```python
from build123d import *

# Parameters (mm, degrees)
SKETCH1_R           = 18.5
SKETCH1_R_2         = 11
BOSS_EXTRUDE1_DEPTH = 3.5
SKETCH2_R           = 4
CUT_EXTRUDE3_DEPTH  = 6.4
CIRPATTERN1_COUNT   = 6
SKETCH3_R           = 4.05
BOSS_EXTRUDE2_DEPTH = 6


with BuildPart() as part:
    # Sketch1 → Boss-Extrude1 (new body, symmetric)
    with BuildSketch(Plane.XY):
        Circle(SKETCH1_R)
        Circle(SKETCH1_R_2, mode=Mode.SUBTRACT)
    extrude(amount=BOSS_EXTRUDE1_DEPTH, both=True)

    # Sketch2 → Cut-Extrude3 (cut)
    with BuildSketch(Plane(origin=(-18.5, -17.193061184, 0), x_dir=(0, -1, 0), z_dir=(1, 0, 0))):
        with Locations((-17.193061184, 0)):
            Circle(SKETCH2_R)
    cut_extrude3 = extrude(amount=CUT_EXTRUDE3_DEPTH, mode=Mode.SUBTRACT)

    # CirPattern1: Cut-Extrude3 ×6 about axis
    cirpattern1_axis = Axis((0, 0, 0), (0, 0, 1))
    for i in range(1, CIRPATTERN1_COUNT):
        add(cut_extrude3.rotate(cirpattern1_axis, i * 360 / CIRPATTERN1_COUNT), mode=Mode.SUBTRACT)

    # Sketch3 → Boss-Extrude2 (add)
    with BuildSketch(Plane(origin=(-12.1, 0, 0), x_dir=(0, -1, 0), z_dir=(-1, 0, 0))):
        Circle(SKETCH3_R)
    extrude(amount=BOSS_EXTRUDE2_DEPTH)


solid = part.part
```
Check sheet for the modelled part. Datum: model origin and axes. Units: mm. A direction names the side the tool comes from. Coordinates: 2 decimals unless noted, no trailing zeros. Write each loop counter-clockwise with the first axis right and the second up, starting at its lowest first coordinate (ties: lowest second). Pieces come first, ordered by that corner, then holes. Notation, with made-up numbers: M 23.5,62 L 79.5,62 A9 cw 79.5,78 Z; hole C 48,20 d7. An arc over 180 degrees is marked long. Use one line per item in the form item = value.
Item 1: Set-up check for faces 1 (the face through (11.11, -11.24, 0.06)), 2 (the face through (11.11, 11.24, -0.06)), 3 (the face through (15, -4, 0)), 4 (the face through (-4.18, 15.24, -0.06)): record each of +Z, -Z, +X, -X, +Y, -Y from which the full face is reachable in a straight line by a thin tool's end or side.
Answer below:
face_1 = -Y
face_2 = +Y
face_3 = +X
face_4 = none
Item 2: Sectioned sample at A-A, the plane y = 0. Record the cut outline in (x, z).
Answer below:
outline = M -18.1,-4.05 L -12.1,-4.05 L -12.1,-3.5 L -11,-3.5 L -11,3.5 L -12.1,3.5 L -12.1,4.05 L -18.1,4.05 Z; M 11,-3.5 L 12.1,-3.5 L 12.1,3.5 L 11,3.5 Z
Item 3: Sectioned sample at C-C, the plane z = -2.25. Record the cut outline in (x, y), and give its area (3 significant figures).
Answer below:
outline = M -18.2,-3.31 A18.5 ccw -11.97,-14.11 L -8.91,-8.83 L -3.19,-12.13 L -6.24,-17.42 A18.5 ccw 6.24,-17.42 L 3.19,-12.13 L 8.91,-8.83 L 11.97,-14.11 A18.5 ccw 18.2,-3.31 L 12.1,-3.31 L 12.1,3.31 L 18.2,3.31 A18.5 ccw 11.97,14.11 L 8.91,8.83 L 3.19,12.13 L 6.24,17.42 A18.5 ccw -6.24,17.42 L -3.19,12.13 L -8.91,8.83 L -11.97,14.11 A18.5 ccw -18.2,3.31 L -18.1,3.31 L -18.1,-3.31 Z; hole C 0,0 d22
area = 485 mm^2
Item 4: Sectioned sample at D-D, the plane y = 5.5. Record the cut outline in (x, z), and give its area (3 significant figures).
Answer below:
outline = M -17.66,-3.5 L -9.53,-3.5 L -9.53,3.5 L -17.66,3.5 Z; M 9.53,-3.5 L 17.66,-3.5 L 17.66,3.5 L 9.53,3.5 Z
area = 114 mm^2
Item 5: Material ranges on L1, parallel to Y at x = 0.5, z = -2.5; L2, parallel to Y at x = 5, z = 1.5; L3, parallel to X at y = 12, z = -2.75, recorded low to high. Write a range as from..to.
Answer below:
L1 = -18.49..-10.99, 10.99..18.49
L2 = -17.81..-16.08, -11.09..-9.8, 9.8..11.09, 16.08..17.81
L3 = -14.08..-10.28, -3.57..3.57, 10.28..14.08
Item 6: Gauge pin test, flat ends, axial feed: pin 1 Ø2 at (y, z) = (0, -1.5) entering from +X; pin 2 Ø5 at (x, y) = (-4.5, -14) entering from +Z; pin 3 Ø6 at (x, y) = (-9.5, 2) entering from +Z. Record the tip position at first contact, or that the pin passes through.
Answer below:
pin_1 = 12.1
pin_2 = 3.5
pin_3 = 4.02
Item 7: Release check for a two-part mould opening along Z. For faces 5 (the face through (-4.18, -15.24, 0.06)), 6 (the face through (-11.11, 11.24, 0.06)), 7 (the face through (8, -8, -3.5)), 8 (the face through (-2.38, -10.74, -0.05)) record: pulls with the +Z half, pulls with the -Z half, needs draft (parallel to the pull), parting line crosses it, or undercut.
Answer below:
face_5 = undercut
face_6 = undercut
face_7 = pulls with the -Z half
face_8 = needs draft
Item 8: Sectioned sample at B-B, the plane x = 0. Record the cut outline in (y, z).
Answer below:
outline = M -18.5,-3.5 L -11,-3.5 L -11,3.5 L -18.5,3.5 Z; M 11,-3.5 L 18.5,-3.5 L 18.5,3.5 L 11,3.5 Z
